Could you check a few things on this model? Use its own coordinates, in mm. A direction names the side the tool comes from. Give positions to 0.01 mm unless a question says otherwise; leave off trailing zeros. Order: outer loops, then holes, each group sorted by start corner. A loop starts at its lowest first (then second) coordinate and runs counter-clockwise, first axis right, second up.
from build123d import *

# Parameters (mm, degrees)
SKETCH2_W           = 20
SKETCH2_H           = 12
BOSS_EXTRUDE1_DEPTH = 4
SKETCH3_W           = 20
SKETCH3_H           = 8
CUT_EXTRUDE1_DEPTH  = 1
SKETCH4_W           = 20
SKETCH4_H           = 0.5
BOSS_EXTRUDE2_DEPTH = 1


with BuildPart() as part:
    # Sketch2 → Boss-Extrude1 (new body)
    with BuildSketch(Plane(origin=(0, 0, 0), x_dir=(1, 0, 0), z_dir=(0, 1, 0))):
        Rectangle(SKETCH2_W, SKETCH2_H)
    extrude(amount=BOSS_EXTRUDE1_DEPTH)

    # Sketch3 → Cut-Extrude1 (cut)
    with BuildSketch(Plane.XZ):
        with Locations((0, 2)):
            Rectangle(SKETCH3_W, SKETCH3_H)
    extrude(amount=-CUT_EXTRUDE1_DEPTH, mode=Mode.SUBTRACT)

    # Sketch4 → Boss-Extrude2 (add)
    with BuildSketch(Plane.XZ.offset(-1)):
        with Locations((0, 5.75)):
            Rectangle(SKETCH4_W, SKETCH4_H)
    extrude(amount=BOSS_EXTRUDE2_DEPTH)


solid = part.part
Item 1: We'd pull the mould along Z, two halves only. Please class faces 3 (the flat face through (-0.1, 0.5, -2)), 4 (the flat face through (0, 0, -4)), 5 (the flat face through (0, 2, 6)): +Z half, -Z half, draft (parallel to the pull), parting line (faces both ways), or undercut.
Findings:
face 3: undercut
face 4: draft
face 5: +Z half
Item 2: Imagine slicing it at A-A on y = 0.45. List the corners of the cut face in (x, z) for me.
Findings:
outline: (-10, -6) - (10, -6) - (10, -2) - (-10, -2) - close; (-10, 5.5) - (10, 5.5) - (10, 6) - (-10, 6) - close
Item 3: For pin 1 (4 mm diameter, centred on x = -6.5, z = 1.5, fed in from -Y), with a flat end and sliding along its axis, tell me the tip position at first contact or that it passes through.
Findings:
pin 1: stops at y = 1
Item 4: Imagine slicing it at B-B on x = 6. List the corners of the cut face in (y, z) for me.
Findings:
outline: (0, -6) - (4, -6) - (4, 6) - (0, 6) - (0, 5.5) - (1, 5.5) - (1, -2) - (0, -2) - close
Item 5: Imagine slicing it at C-C on z = 3.75. List the corners of the cut face in (x, y) for me, then the cut area to 3 significant figures.
Findings:
outline: (-10, 1) - (10, 1) - (10, 4) - (-10, 4) - close
area: 60.0 mm2
Item 6: For faces 1 (the flat face through (0, 2, -6)), 2 (the flat face through (0, 1, 2)), which set-ups out of +Z, -Z, +X, -X, +Y, -Y let a thin tool reach every point of the face, with its end or its side?
Findings:
face 1: -Z, +X, -X, +Y, -Y
face 2: +X, -X, -Y
Item 7: Please list where these lines run through material, in increasing order: line 1 along Z through (x, y) = (0.5, 0.4); line 2 along Y through (x, z) = (1.75, 0.25).
Findings:
line 1: z = -6 to -2, 5.5 to 6
line 2: y = 1 to 4
